Here's how the part is built. I have some questions about the finished solid (model axes, mm). Round coordinates to 2 decimals unless told otherwise and drop trailing zeros. Order: outer loops, then holes, each group sorted by start corner. A loop starts at its lowest first (then second) coordinate and runs counter-clockwise, first axis right, second up. Notation, with made-up numbers: (53.5, 41.5) -> (111.5, 41.5) arc R25 cw to (111.5, 66.5) -> close; hole circle Ø1 at (9, -12.5). An arc over 180 degrees is marked (long way). One line per item, written item: value.
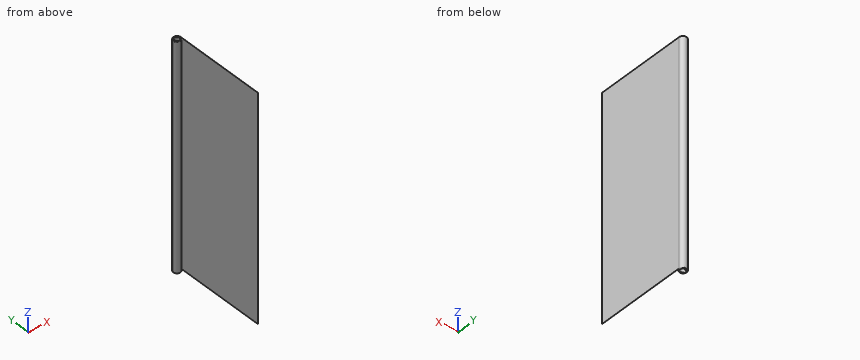
```python
from build123d import *

# Parameters (mm, degrees)
SKETCH_2_W = 0.5
SKETCH_2_H = 1500


with BuildPart() as part:
    # 扫描1: sweep along a path in 草图1
    with BuildLine(Plane.XY) as sweep_1_path:
        Line((25, -600), (25, 0))
        ThreePointArc((25, 0), (0, 25), (-25, 0))
        ThreePointArc((-25, 0), (-1.25, -23.75), (22.5, 0))
        ThreePointArc((22.5, 0), (0, 22.5), (-22.5, 0))
        ThreePointArc((-22.5, 0), (-1.25, -21.25), (20, 0))
        ThreePointArc((20, 0), (0, 20), (-20, 0))
        ThreePointArc((-20, 0), (-1.25, -18.75), (17.5, 0))
        ThreePointArc((17.5, 0), (0, 17.5), (-17.5, 0))
        ThreePointArc((-17.5, 0), (-1.25, -16.25), (15, 0))
        ThreePointArc((15, 0), (0, 15), (-15, 0))
    # 草图2 → 扫描1 (sweep)
    with BuildSketch(Plane(origin=(0, -600, 0), x_dir=(1, 0, 0), z_dir=(0, 1, 0))):
        with Locations((25, 0)):
            Rectangle(SKETCH_2_W, SKETCH_2_H)
    sweep(path=sweep_1_path.line)


solid = part.part
```
Q1. I want a section at C-C on x = 6. Give the number of separate pieces and of enclosed holes in the cut face, then the cut area to 3 significant figures.
Answers:
separate pieces: 9
enclosed holes: 0
area: 7,190 mm2
Q2. I want a section at B-B on y = -279.5. Write out the boundary of the cut face in (x, z), then the cut area to 3 significant figures.
Answers:
outline: (24.75, -750) -> (25.25, -750) -> (25.25, 750) -> (24.75, 750) -> close
area: 750 mm2
Q3. For P1, Ø3, axis at y = -116.5, z = 159, coming from the -X side; P2, Ø2, axis at x = -1, z = -331.5, coming from the +Y side; P3, Ø8, axis at x = -11.5, z = 360, coming from the -Y side, each with a flat end and sliding along its axis, tell me the tip position at first contact or that it passes through.
Answers:
P1: x = 24.75
P2: y = 25.25
P3: y = -23.17
Q4. I need wall thicknesses on line 1 along X through (y, z) = (-394, 243.5); line 2 along Y through (x, z) = (18, -440). Which ranges of each line are inside material? Lowest first, please.
Answers:
line 1: 24.75 to 25.25
line 2: -14.33 to -13.48, -9.58 to -8.39, 8.13 to 9.28, 13.08 to 13.91, 16.99 to 17.71
Q5. I want a section at A-A on z = -561.5. Write out the boundary of the cut face in (x, y).
Answers:
outline: (-25.25, 0) arc R24 ccw to (22.75, 0) arc R22.75 ccw to (-22.75, 0) arc R21.5 ccw to (20.25, 0) arc R20.25 ccw to (-20.25, 0) arc R19 ccw to (17.75, 0) arc R17.75 ccw to (-17.75, 0) arc R16.5 ccw to (15.25, 0) arc R15.25 ccw to (-15.25, 0) -> (-14.75, 0) arc R14.75 cw to (14.75, 0) arc R16 cw to (-17.25, 0) arc R17.25 cw to (17.25, 0) arc R18.5 cw to (-19.75, 0) arc R19.75 cw to (19.75, 0) arc R21 cw to (-22.25, 0) arc R22.25 cw to (22.25, 0) arc R23.5 cw to (-24.75, 0) arc R24.75 cw to (24.75, 0) -> (24.75, -600) -> (25.25, -600) -> (25.25, 0) arc R25.25 ccw to start
